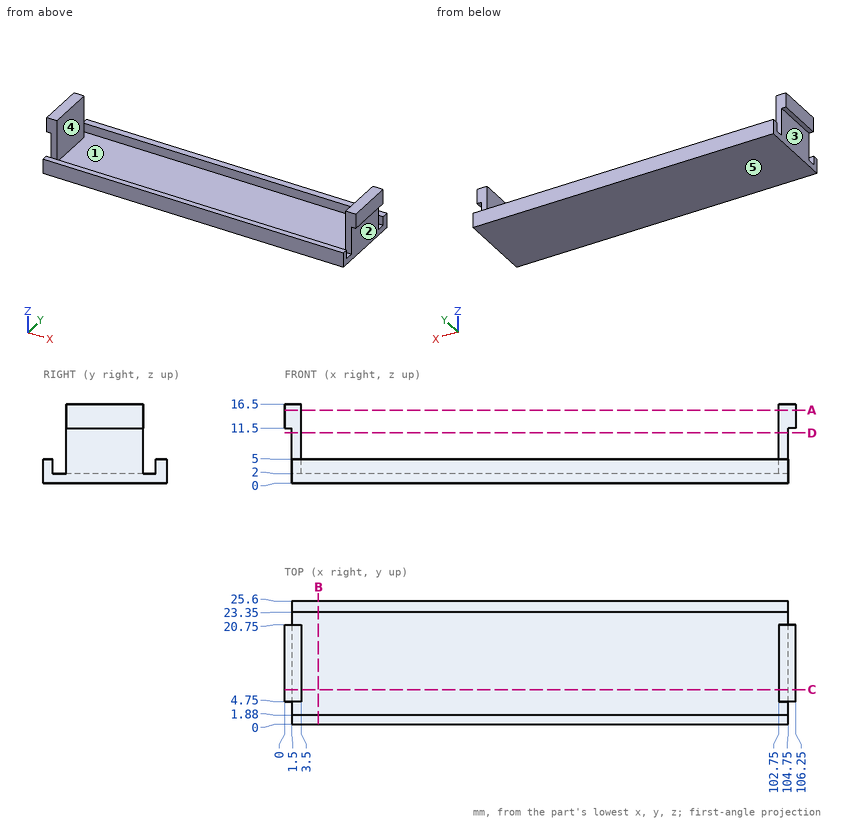
The figure shows three views and two pictorial views of one solid part (mm, origin at its lowest corner). Answer the questions. A direction names the side the tool comes from. Coordinates: 2 decimals unless noted, no trailing zeros. Loops run counter-clockwise (first coordinate to the right, second up) from the corner with the lowest first, then second, coordinate; pieces in that order, holes last.
1) Find section A-A on z = 15.25. Write down the section's boundary in (x, y).
2) Find section D-D on z = 10.5. Write down the section's boundary in (x, y).
3) Find the intervals of material crossed by L1, parallel to X at y = 6.25, z = 6.75; L2, parallel to Y at x = 13.5, z = 4; L3, parallel to X at y = 8.5, z = 15.5, in increasing order.
4) Find section B-B on x = 7. Write down the section's boundary in (y, z), then the cut area to 3 significant figures.
5) A tool of negligible diameter and unlimited length cuts with its end or side. For the marked faces 4 and 5, from which of +Z, -Z, +X, -X, +Y, -Y can it reach the whole face along a straight path? Write none if from no direction.
6) Flat-ended cylindrical pins translate along their axes: pin 1 Ø4 at (x, z) = (105.5, 6.5) entering from +Y; pin 2 Ø3 at (y, z) = (23, 5) entering from -X; pin 3 Ø2.5 at (x, y) = (35, 24.5) entering from +Z; pin 4 Ø1 at (x, y) = (43.5, 6) entering from +Z. Find the tip coordinate at first contact, or state that the pin passes through.
7) Find section C-C on y = 7.25. Write down the section's boundary in (x, z).
8) Determine the mould class of the marked faces 1, 2 and 3 for opening direction X: pulls with the +X half, pulls with the -X half, needs draft (parallel to the pull), parting line crosses it, or undercut.
Values:
1. outline: (0, 4.75) - (3.5, 4.75) - (3.5, 20.75) - (0, 20.75) - close; (102.75, 4.75) - (106.25, 4.75) - (106.25, 20.75) - (102.75, 20.75) - close
2. outline: (1.5, 4.75) - (3.5, 4.75) - (3.5, 20.75) - (1.5, 20.75) - close; (102.75, 4.75) - (104.75, 4.75) - (104.75, 20.75) - (102.75, 20.75) - close
3. L1: x = 1.5 to 3.5, 102.75 to 104.75
3. L2: y = 0 to 1.88, 23.35 to 25.6
3. L3: x = 0 to 3.5, 102.75 to 106.25
4. outline: (0, 0) - (25.6, 0) - (25.6, 5) - (23.35, 5) - (23.35, 2) - (1.88, 2) - (1.88, 5) - (0, 5) - close
4. area: 63.6 mm2
5. face 4: +Z
5. face 5: -Z, +X, -X, +Y, -Y
6. pin 1: stops at y = 25.6
6. pin 2: stops at x = 1.5
6. pin 3: stops at z = 5
6. pin 4: stops at z = 2
7. outline: (0, 11.5) - (1.5, 11.5) - (1.5, 0) - (104.75, 0) - (104.75, 11.5) - (106.25, 11.5) - (106.25, 16.5) - (102.75, 16.5) - (102.75, 2) - (3.5, 2) - (3.5, 16.5) - (0, 16.5) - close
8. face 1: undercut
8. face 2: pulls with the +X half
8. face 3: pulls with the -X half
